Verification items for the finished model (mm, model axes). Face numbers are marked on the shaded views. A direction names the side the tool comes from. Round coordinates to 2 decimals unless told otherwise and drop trailing zeros. Write each loop counter-clockwise with the first axis right and the second up, starting at its lowest first coordinate (ties: lowest second). Pieces come first, ordered by that corner, then holes.
from build123d import *

# Parameters (mm, degrees)
BOSS_EXTRUDE1_DEPTH = 70
SKETCH2_W           = 50
SKETCH2_H           = 74.667138355
CUT_EXTRUDE1_DEPTH  = 48
BOSS_EXTRUDE2_DEPTH = 75
BOSS_EXTRUDE3_DEPTH = 40
SKETCH5_R           = 16
CUT_EXTRUDE2_DEPTH  = 70


with BuildPart() as part:
    # Sketch1 → Boss-Extrude1 (new body)
    with BuildSketch(Plane(origin=(0, 0, 0), x_dir=(1, 0, 0), z_dir=(0, 1, 0))):
        with BuildLine():
            Line((-46.249324319, -19), (46.249324319, -19))
            ThreePointArc((46.249324319, -19), (0, 50), (-46.249324319, -19))
        make_face()
    extrude(amount=BOSS_EXTRUDE1_DEPTH)

    # Sketch2 → Cut-Extrude1 (cut)
    with BuildSketch(Plane(origin=(0, 70, 0), x_dir=(1, 0, 0), z_dir=(0, 1, 0))):
        with Locations((0, 18.333569178)):
            Rectangle(SKETCH2_W, SKETCH2_H)
    extrude(amount=-CUT_EXTRUDE1_DEPTH, mode=Mode.SUBTRACT)

    # Sketch3 → Boss-Extrude2 (add)
    with BuildSketch(Plane.XZ):
        with BuildLine():
            Line((32.330326321, 19), (-32.330326321, 19))
            ThreePointArc((-32.330326321, 19), (0, -37.5), (32.330326321, 19))
        make_face()
    extrude(amount=BOSS_EXTRUDE2_DEPTH)

    # Sketch4 → Boss-Extrude3 (add)
    with BuildSketch(Plane.XZ.offset(75)):
        with BuildLine():
            Line((-37.016888038, -6), (37.016888038, -6))
            ThreePointArc((37.016888038, -6), (0, -37.5), (-37.016888038, -6))
        make_face()
    extrude(amount=BOSS_EXTRUDE3_DEPTH)

    # Sketch5 → Cut-Extrude2 (cut, through all)
    with BuildSketch(Plane.XY.offset(19)):
        with Locations((0, -42)):
            Circle(SKETCH5_R)
    extrude(amount=-CUT_EXTRUDE2_DEPTH, mode=Mode.SUBTRACT)


solid = part.part
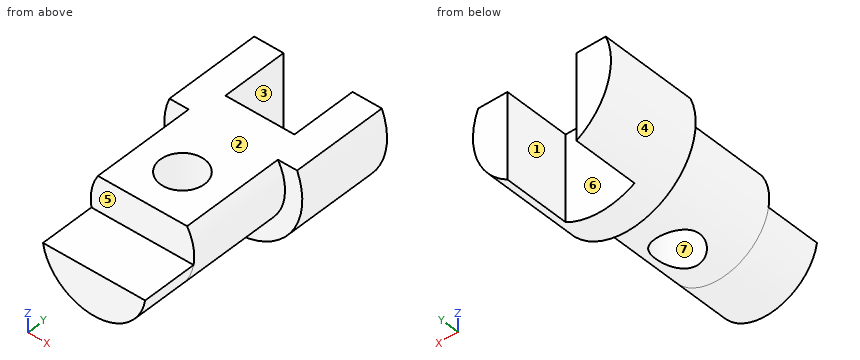
Q1. Depth check by flat-ended pin: P1, Ø12, axis at x = -5, z = 6, coming from the -Y side; P2, Ø2, axis at y = 39.5, z = 2, coming from the -X side; P3, Ø4, axis at x = -11.5, z = -36, coming from the +Y side. Enter the tip coordinate at first touch or a pass-through.
Recorded:
P1: stops at y = -75
P2: stops at x = -49.99
P3: stops at y = 22
Q2. Tool access check on the marked faces 5, 6 and 7. Record the directions out of +Z, -Z, +X, -X, +Y, -Y that give a thin tool (end or side, any length) a straight path to the whole face; none if there is none.
Recorded:
face 5: +Z, +X, -X, -Y
face 6: +Z, -Z, +Y
face 7: +Z, -Z
Q3. Sectioned sample at B-B (y = 24). Enter the section's corners in (x, z).
Recorded:
outline: (-46.25, 19) arc R50 ccw to (-25, -43.3) - (-25, 19) - close; (25, -43.3) arc R50 ccw to (46.25, 19) - (25, 19) - close
Q4. Sectioned sample at D-D (x = 18). Enter the section's corners in (y, z), plus the area to 3 significant figures.
Recorded:
outline: (-115, -32.9) - (0, -32.9) - (0, -46.65) - (22, -46.65) - (22, 19) - (-75, 19) - (-75, -6) - (-115, -6) - close
area: 6,410 mm2
Q5. Material ranges on line 1 along Y through (x, z) = (0, -23); line 2 along Y through (x, z) = (-1, 14); line 3 along X through (y, z) = (-42, 1), recorded low to high.
Recorded:
line 1: y = -115 to -58, -26 to 22
line 2: y = -75 to -57.97, -26.03 to 22
line 3: x = -37.49 to -16, 16 to 37.49
Q6. Sectioned sample at C-C (z = 0). Enter the section's corners in (x, y), plus the area to 3 significant figures.
Recorded:
outline: (-50, 0) - (-37.5, 0) - (-37.5, -75) - (37.5, -75) - (37.5, 0) - (50, 0) - (50, 70) - (25, 70) - (25, 22) - (-25, 22) - (-25, 70) - (-50, 70) - close; hole circle Ø32 at (0, -42)
area: 9,420 mm2
Q7. Release check for a two-part mould opening along X. For the marked faces 1, 2, 3 and 4 record: released by +X, released by -X, zero draft, split by the parting line, or undercut.
Recorded:
face 1: undercut
face 2: zero draft
face 3: undercut
face 4: split by the parting line
Q8. Sectioned sample at A-A (x = 0). Enter the section's corners in (y, z), plus the area to 3 significant figures.
Recorded:
outline: (-115, -37.5) - (-58, -37.5) - (-58, 19) - (-75, 19) - (-75, -6) - (-115, -6) - close; (-26, -37.5) - (0, -37.5) - (0, -50) - (22, -50) - (22, 19) - (-26, 19) - close
area: 5,210 mm2
